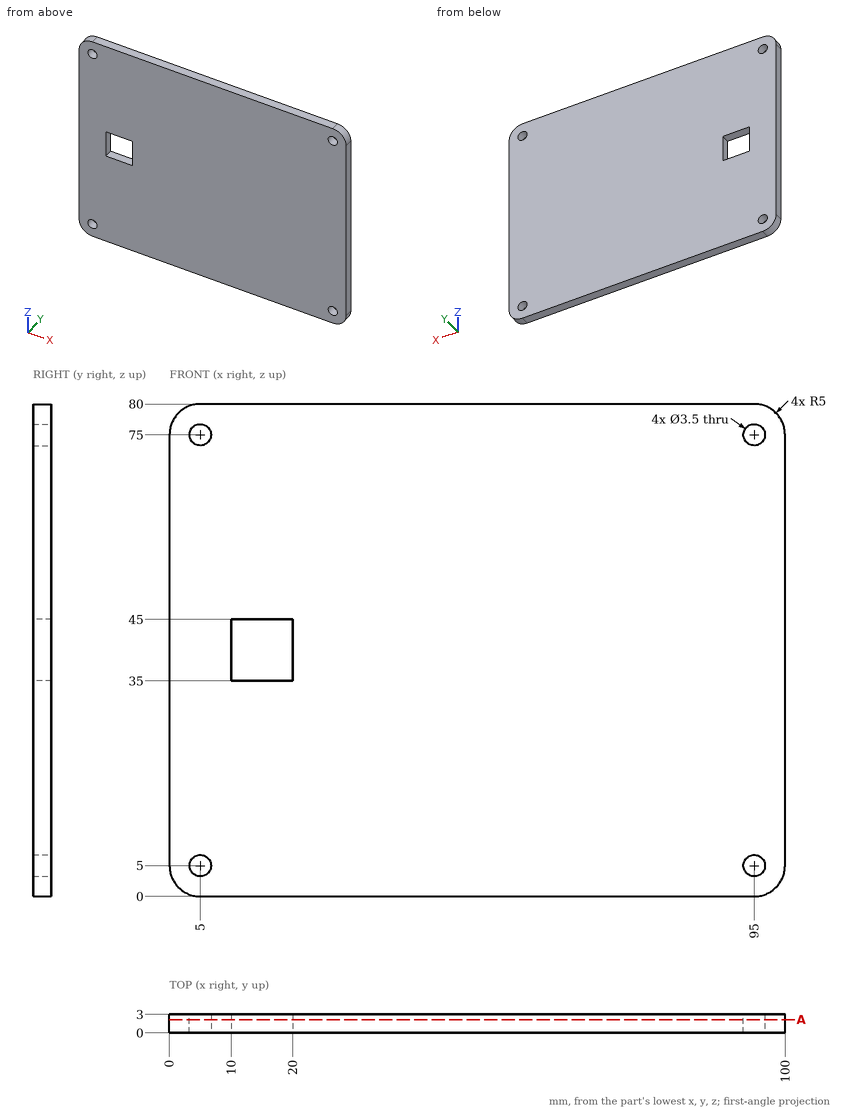
Answer from the drawing. Dimensions are ordinates in mm from the lowest x, y and z of the part. Coordinates: 2 decimals unless noted, no trailing zeros. Write each loop counter-clockwise with the first axis right and the second up, starting at its lowest first coordinate (ties: lowest second). Pieces come first, ordered by that corner, then holes. Notation, with made-up numbers: (0.5, 76) - (41.5, 76) arc R18 cw to (41.5, 93) - close; hole circle Ø1 at (33.25, 37). An arc over 180 degrees is marked (long way). Return JSON: item names as keys, results as strings.
1. This flat-tipped pin is pushed along its axis until it touches: pin 1 Ø2 at (x, z) = (5, 5) entering from -Y. Where does it stop, or does it pass through?
Final values:
{"pin 1": "through"}
2. Consider line 1 along X through (y, z) = (1.1, 5); line 2 along Z through (x, y) = (95, 1.6); line 3 along Z through (x, y) = (14, 1.85). Determine where each line is inside the solid, lowest interval first.
Final values:
{"line 1": "0 to 3.25, 6.75 to 93.25, 96.75 to 100", "line 2": "0 to 3.25, 6.75 to 73.25, 76.75 to 80", "line 3": "0 to 35, 45 to 80"}
3. The part is cut by section A-A on y = 2.15. Determine the outline of the cut face in (x, z), then the cut area to 3 significant figures.
Final values:
{"outline": "(0, 5) arc R5 ccw to (5, 0) - (95, 0) arc R5 ccw to (100, 5) - (100, 75) arc R5 ccw to (95, 80) - (5, 80) arc R5 ccw to (0, 75) - close; hole circle Ø3.5 at (5, 5); hole circle Ø3.5 at (5, 75); hole (10, 35) - (20, 35) - (20, 45) - (10, 45) - close; hole circle Ø3.5 at (95, 5); hole circle Ø3.5 at (95, 75)", "area": "7,840 mm^2"}
